from build123d import *

# Parameters (mm, degrees)
F0_W      = 2
F0_H      = 2
F1_DEPTH  = 3
F0_H_2    = 14
F0_W_2    = 14
F0_W_3    = 11
F2_DEPTH  = 2
F0_R      = 2.5
F3_DEPTH  = 4
F0_R_2    = 1.5
F0_R_3    = 0.95
F4_DEPTH  = 20
F5_DEPTH  = 17
F6_DEPTH  = 17
F7_DEPTH  = 17
F8_DEPTH  = 17
F0_W_4    = 6
F0_H_3    = 6
F9_DEPTH  = 2
F0_H_4    = 3
F10_DEPTH = 20
F0_W_5    = 3
F0_W_6    = 5
F0_W_7    = 1.1521804929
F0_H_5    = 5
F0_R_4    = 1.75
F0_R_5    = 1
F0_W_8    = 0.8478195071
F11_DEPTH = 2
F0_H_6    = 1
F12_DEPTH = 4
F0_W_9    = 2.5
F13_DEPTH = 4
F14_DEPTH = 2
F15_DEPTH = 2
F16_DEPTH = 0.5


# Not quite as in the source:
# - a feature names something its author has since deleted; it is built from what else it names


with BuildPart() as f1:
    # F0 (on Front) → F1 (new body)
    with BuildSketch(Plane.XZ):
        Polygon((16, 1), (16, 2), (2, 2), (1, 2), (-1, 2), (-1, 10), (-1, 16), (-2, 16), (-2, 2), (-4, 2), (-4, 16), (-5, 16), (-5, 2), (-16, 2), (-16, 1), (-5, 1), (-5, -1), (-16, -1), (-16, -2), (-5, -2), (-5, -16), (-4, -16), (-4, -2), (-2, -2), (-2, -16), (-1, -16), (-1, -2), (1, -2), (1, -16), (2, -16), (2, -2), (16, -2), (16, -1), (2, -1), (2, 1), align=None)
        with Locations((-3, 0)):
            Rectangle(F0_W, F0_H, mode=Mode.SUBTRACT)
        Rectangle(F0_W, F0_H, mode=Mode.SUBTRACT)
    extrude(amount=-F1_DEPTH)

    # F0 (on Front) → F2 (join)
    with BuildSketch(Plane.XZ):
        Polygon((16, 2), (16, 10.1685791543), (16, 11), (11, 11), (9.8478195071, 11), (9.8478195071, 10.2023985237), (9.8478195071, 10), (7.6956390142, 10), (7.6956390142, 7.9433578615), (7.6956390142, 6.0566421385), (7.6956390142, 4), (4.8478195071, 4), (2, 4), (2, 6.0566421385), (2, 7.9433578615), (2, 10), (-0.1521804929, 10), (-1, 10), (-1, 2), (1, 2), (2, 2), align=None)
        with Locations((-3, 9)):
            Rectangle(F0_W, F0_H_2)
        Polygon((16, -11), (16, -2), (2, -2), (2, -16), (11, -16), (11, -11), align=None)
        with Locations((9, 0)):
            Rectangle(F0_W_2, F0_H)
        with Locations((-10.5, 0)):
            Rectangle(F0_W_3, F0_H)
        Polygon((-11, -11), (-11, -16), (-5, -16), (-5, -2), (-16, -2), (-16, -11), align=None)
        with Locations((-3, -9)):
            Rectangle(F0_W, F0_H_2)
        with Locations((0, -9)):
            Rectangle(F0_W, F0_H_2)
        Polygon((-5, 2), (-5, 16), (-11, 16), (-11, 11), (-16, 11), (-16, 10), (-10, 10), (-10, 4), (-16, 4), (-16, 2), align=None)
        with Locations((-3, 0)):
            Rectangle(F0_W, F0_H)
        Rectangle(F0_W, F0_H)
    extrude(amount=-F2_DEPTH)

    # F0 (on Front) → F3 (join)
    with BuildSketch(Plane.XZ):
        Polygon((11, 11), (16, 11), (17, 11), (17, 13), (17, 14), (17, 17), (14, 17), (11, 17), (11, 16), align=None)
        with Locations((14, 14)):
            Circle(F0_R, mode=Mode.SUBTRACT)
        Polygon((-11, 16), (-11, 17), (-14, 17), (-17, 17), (-17, 14), (-17, 11), (-16, 11), (-11, 11), align=None)
        with Locations((-14, 14)):
            Circle(F0_R, mode=Mode.SUBTRACT)
        Polygon((-14, -17), (-11, -17), (-11, -16), (-11, -11), (-16, -11), (-17, -11), (-17, -14), (-17, -17), align=None)
        with Locations((-14, -14)):
            Circle(F0_R, mode=Mode.SUBTRACT)
        Polygon((17, -11), (16, -11), (11, -11), (11, -16), (11, -17), (14, -17), (17, -17), (17, -14), (17, -13), align=None)
        with Locations((14, -14)):
            Circle(F0_R, mode=Mode.SUBTRACT)
    extrude(amount=-F3_DEPTH)

    # F0 (on Front) → F4 (join)
    with BuildSketch(Plane.XZ):
        with Locations((14, 14)):
            Circle(F0_R)
        with Locations((14, 14)):
            Circle(F0_R_2, mode=Mode.SUBTRACT)
        with Locations((14, 14)):
            Circle(F0_R_2)
        with Locations((14, 14)):
            Circle(F0_R_3, mode=Mode.SUBTRACT)
        with Locations((-14, 14)):
            Circle(F0_R)
        with Locations((-14, 14)):
            Circle(F0_R_2, mode=Mode.SUBTRACT)
        with Locations((-14, 14)):
            Circle(F0_R_2)
        with Locations((-14, 14)):
            Circle(F0_R_3, mode=Mode.SUBTRACT)
        with Locations((-14, -14)):
            Circle(F0_R)
        with Locations((-14, -14)):
            Circle(F0_R_2, mode=Mode.SUBTRACT)
        with Locations((-14, -14)):
            Circle(F0_R_2)
        with Locations((-14, -14)):
            Circle(F0_R_3, mode=Mode.SUBTRACT)
        with Locations((14, -14)):
            Circle(F0_R)
        with Locations((14, -14)):
            Circle(F0_R_2, mode=Mode.SUBTRACT)
        with Locations((14, -14)):
            Circle(F0_R_2)
        with Locations((14, -14)):
            Circle(F0_R_3, mode=Mode.SUBTRACT)
    extrude(amount=-F4_DEPTH)

    # F0 (on Front) → F5 (cut)
    with BuildSketch(Plane.XZ):
        with Locations((-14, 14)):
            Circle(F0_R_2)
        with Locations((-14, 14)):
            Circle(F0_R_3, mode=Mode.SUBTRACT)
    extrude(amount=-F5_DEPTH, mode=Mode.SUBTRACT)

    # F0 (on Front) → F6 (cut)
    with BuildSketch(Plane.XZ):
        with Locations((14, 14)):
            Circle(F0_R_2)
        with Locations((14, 14)):
            Circle(F0_R_3, mode=Mode.SUBTRACT)
    extrude(amount=-F6_DEPTH, mode=Mode.SUBTRACT)

    # F0 (on Front) → F7 (cut)
    with BuildSketch(Plane.XZ):
        with Locations((-14, -14)):
            Circle(F0_R_2)
        with Locations((-14, -14)):
            Circle(F0_R_3, mode=Mode.SUBTRACT)
    extrude(amount=-F7_DEPTH, mode=Mode.SUBTRACT)

    # F0 (on Front) → F8 (cut)
    with BuildSketch(Plane.XZ):
        with Locations((14, -14)):
            Circle(F0_R_2)
        with Locations((14, -14)):
            Circle(F0_R_3, mode=Mode.SUBTRACT)
    extrude(amount=-F8_DEPTH, mode=Mode.SUBTRACT)

    # F0 (on Front) → F9 (join)
    with BuildSketch(Plane.XZ):
        with Locations((-13, 7)):
            Rectangle(F0_W_4, F0_H_3)
    extrude(amount=-F9_DEPTH)

    # F0 (on Front) → F10, piece 6 (join)
    with BuildSketch(Plane.XZ):
        with Locations((18, 18)):
            Rectangle(F0_W, F0_H)
        with Locations((18, 15.5)):
            Rectangle(F0_W, F0_H_4)
        with Locations((15.5, 18)):
            Rectangle(F0_W_5, F0_H)
        Polygon((9.8478195071, 17), (11, 17), (14, 17), (14, 19), (7.3478195071, 19), (7.3478195071, 17), align=None)
        with Locations((4.8478195071, 18)):
            Rectangle(F0_W_6, F0_H)
        Polygon((-0.1521804929, 17), (2.3478195071, 17), (2.3478195071, 19), (-14, 19), (-14, 17), (-11, 17), align=None)
        with Locations((-15.5, 18)):
            Rectangle(F0_W_5, F0_H)
        with Locations((-18, 18)):
            Rectangle(F0_W, F0_H)
        with Locations((-18, 15.5)):
            Rectangle(F0_W, F0_H_4)
        Polygon((-19, -14), (-17, -14), (-17, -11), (-17, -2), (-17, -1), (-17, 1), (-17, 2), (-17, 11), (-17, 14), (-19, 14), align=None)
        Polygon((17, 13), (17, 11), (17, 10), (19, 10), (19, 13), align=None)
        Polygon((17, -10), (17, -11), (17, -13), (19, -13), (19, -10), align=None)
        with Locations((18, -15.5)):
            Rectangle(F0_W, F0_H_4)
        with Locations((18, -18)):
            Rectangle(F0_W, F0_H)
        with Locations((15.5, -18)):
            Rectangle(F0_W_5, F0_H)
        Polygon((14, -17), (11, -17), (-11, -17), (-14, -17), (-14, -19), (14, -19), align=None)
        with Locations((-15.5, -18)):
            Rectangle(F0_W_5, F0_H)
        with Locations((-18, -18)):
            Rectangle(F0_W, F0_H)
        with Locations((-18, -15.5)):
            Rectangle(F0_W, F0_H_4)
    extrude(amount=-F10_DEPTH)

    # F0 (on Front) → F11 (join)
    with BuildSketch(Plane.XZ):
        with Locations((10.4239097536, 13.5)):
            Rectangle(F0_W_7, F0_H_5)
        with BuildLine():
            Line((7.6956390142, 7.9433578615), (7.6956390142, 10))
            Line((7.6956390142, 10), (4.8478195071, 10))
            ThreePointArc((4.8478195071, 10), (6.6042258404, 9.4320848653), (7.6956390142, 7.9433578615))
        make_face()
        with BuildLine():
            ThreePointArc((7.6956390142, 7.9433578615), (6.6042258404, 9.4320848653), (4.8478195071, 10))
            ThreePointArc((4.8478195071, 10), (3.0914131738, 9.4320848653), (2, 7.9433578615))
            Line((2, 7.9433578615), (2, 6.0566421385))
            ThreePointArc((2, 6.0566421385), (3.0914131738, 4.5679151347), (4.8478195071, 4))
            ThreePointArc((4.8478195071, 4), (6.6042258404, 4.5679151347), (7.6956390142, 6.0566421385))
            Line((7.6956390142, 6.0566421385), (7.6956390142, 7.9433578615))
        make_face()
        with Locations((4.8478195071, 7)):
            Circle(F0_R_4, mode=Mode.SUBTRACT)
        with BuildLine():
            Line((7.6956390142, 4), (7.6956390142, 6.0566421385))
            ThreePointArc((7.6956390142, 6.0566421385), (6.6042258404, 4.5679151347), (4.8478195071, 4))
            Line((4.8478195071, 4), (7.6956390142, 4))
        make_face()
        with Locations((4.8478195071, 7)):
            Circle(F0_R_4)
        with Locations((4.8478195071, 7)):
            Circle(F0_R_5, mode=Mode.SUBTRACT)
        with BuildLine():
            ThreePointArc((4.8478195071, 4), (3.0914131738, 4.5679151347), (2, 6.0566421385))
            Line((2, 6.0566421385), (2, 4))
            Line((2, 4), (4.8478195071, 4))
        make_face()
        with BuildLine():
            Line((4.8478195071, 10), (2, 10))
            Line((2, 10), (2, 7.9433578615))
            ThreePointArc((2, 7.9433578615), (3.0914131738, 9.4320848653), (4.8478195071, 10))
        make_face()
        with Locations((-0.5760902464, 13)):
            Rectangle(F0_W_8, F0_H_3)
    extrude(amount=-F11_DEPTH)



with BuildPart() as f10:
    # F0 (on Front) → F10 (new body)
    with BuildSketch(Plane.XZ):
        with Locations((18, 7.5)):
            Rectangle(F0_W, F0_H_4)
    extrude(amount=-F10_DEPTH)


with BuildPart() as f10b:
    # F0 (on Front) → F10, piece 2 (new body)
    with BuildSketch(Plane.XZ):
        with Locations((18, 3.5)):
            Rectangle(F0_W, F0_H_4)
    extrude(amount=-F10_DEPTH)


with BuildPart() as f10c:
    # F0 (on Front) → F10, piece 3 (new body)
    with BuildSketch(Plane.XZ):
        Polygon((19, 1), (17, 1), (17, 0), (17, -1), (19, -1), (19, 0), align=None)
    extrude(amount=-F10_DEPTH)


with BuildPart() as f10d:
    # F0 (on Front) → F10, piece 4 (new body)
    with BuildSketch(Plane.XZ):
        with Locations((18, -3.5)):
            Rectangle(F0_W, F0_H_4)
    extrude(amount=-F10_DEPTH)


with BuildPart() as f10e:
    # F0 (on Front) → F10, piece 5 (new body)
    with BuildSketch(Plane.XZ):
        with Locations((18, -7.5)):
            Rectangle(F0_W, F0_H_4)
    extrude(amount=-F10_DEPTH)


with BuildPart() as f1_1:
    add(f1.part)

    add(f10.part)  # F12 merges F10

    add(f10b.part)  # F12 merges F10b

    add(f10c.part)  # F12 merges F10c

    add(f10d.part)  # F12 merges F10d

    add(f10e.part)  # F12 merges F10e
    # F0 (on Front) → F12 (join)
    with BuildSketch(Plane.XZ):
        Polygon((16, 11), (16, 10.1685791543), (16, 2), (16, 1), (16, -1), (16, -2), (16, -11), (17, -11), (17, -10), (17, -9), (17, -6), (17, -5), (17, -2), (17, -1), (17, 0), (17, 1), (17, 2), (17, 5), (17, 6), (17, 9), (17, 10), (17, 11), align=None)
        with Locations((4.8478195071, 16.5)):
            Rectangle(F0_W_6, F0_H_6)
        Polygon((11, -16), (2, -16), (1, -16), (-1, -16), (-2, -16), (-4, -16), (-5, -16), (-11, -16), (-11, -17), (11, -17), align=None)
        Polygon((-2, 16), (-1, 16), (-0.1521804929, 16), (-0.1521804929, 17), (-11, 17), (-11, 16), (-5, 16), (-4, 16), align=None)
        Polygon((-16, 1), (-16, 2), (-16, 4), (-16, 10), (-16, 11), (-17, 11), (-17, 2), (-17, 1), (-17, -1), (-17, -2), (-17, -11), (-16, -11), (-16, -2), (-16, -1), align=None)
    extrude(amount=-F12_DEPTH)

    # F0 (on Front) → F13 (join)
    with BuildSketch(Plane.XZ):
        with Locations((10.4239097536, 16.5)):
            Rectangle(F0_W_7, F0_H_6)
        with Locations((8.5978195071, 16.5)):
            Rectangle(F0_W_9, F0_H_6)
        Polygon((2, 16), (2.3478195071, 16), (2.3478195071, 17), (-0.1521804929, 17), (-0.1521804929, 16), (1, 16), align=None)
    extrude(amount=-F13_DEPTH)

    # F0 (on Front) → F14 (cut)
    with BuildSketch(Plane.XZ):
        Polygon((2, 16), (2.3478195071, 16), (2.3478195071, 17), (-0.1521804929, 17), (-0.1521804929, 16), (1, 16), align=None)
    extrude(amount=-F14_DEPTH, mode=Mode.SUBTRACT)

    # F0 (on Front) → F15 (cut)
    with BuildSketch(Plane.XZ):
        with Locations((8.5978195071, 16.5)):
            Rectangle(F0_W_9, F0_H_6)
    extrude(amount=-F15_DEPTH, mode=Mode.SUBTRACT)

    # F0 (on Front) → F16 (cut)
    with BuildSketch(Plane.XZ):
        with Locations((4.8478195071, 7)):
            Circle(F0_R_4)
        with Locations((4.8478195071, 7)):
            Circle(F0_R_5, mode=Mode.SUBTRACT)
    extrude(amount=-F16_DEPTH, mode=Mode.SUBTRACT)


solid = f1_1.part
Geometry: final body of the model. Coordinates: model frame, mm. A direction names the side the tool comes from. Round coordinates to 2 decimals unless told otherwise and drop trailing zeros. Order: outer loops, then holes, each group sorted by start corner. A loop starts at its lowest first (then second) coordinate and runs counter-clockwise, first axis right, second up.
Q1. Access query for faces 3 (the face through (-3, 2.5, -2)), 4 (the face through (18, 10, 14)), 5 (the face through (1.1, 2, 16.5)), 6 (the face through (18, 20, -11)), 7 (the face through (19, 10, 11)). Directions: +Z, -Z, +X, -X, +Y, -Y. A direction counts if a zero-diameter tool reaches every point of the face in a straight line with its end or side. Return the directions, or none.
Result sheet:
face 3: +Y
face 4: +X, +Y, -Y
face 5: -Y
face 6: +Z, -Z, +X, -X, +Y
face 7: +Z, -Z, +X, +Y, -Y
Q2. Section A-A, the plane z = 7. Output: boundary loops of the cut face in (x, y), and give its area (3 significant figures).
Result sheet:
outline: (-19, 0) - (3.1, 0) - (3.1, 0.5) - (3.85, 0.5) - (3.85, 2) - (-1, 2) - (-1, 3) - (-2, 3) - (-2, 2) - (-4, 2) - (-4, 3) - (-5, 3) - (-5, 2) - (-16, 2) - (-16, 4) - (-17, 4) - (-17, 20) - (-19, 20) - close; (5.85, 0.5) - (6.6, 0.5) - (6.6, 0) - (19, 0) - (19, 20) - (17, 20) - (17, 4) - (16, 4) - (16, 2) - (5.85, 2) - close
area: 149 mm2
Q3. Pin query (flat end, axial travel): pin 1 (2.5 mm diameter, centred on x = 14, z = 14, fed in from -Y); pin 2 (0.8 mm diameter, centred on y = 1.5, z = -5.5, fed in from +X); pin 3 (1.6 mm diameter, centred on x = 0, z = 0, fed in from +Y). Return the tip coordinate at first contact, or that it passes through.
Result sheet:
pin 1: stops at y = 17
pin 2: stops at x = 17
pin 3: stops at y = 2
Q4. Section C-C, the plane x = 10.5. Output: boundary loops of the cut face in (y, z).
Result sheet:
outline: (0, -19) - (20, -19) - (20, -17) - (4, -17) - (4, -16) - (2, -16) - (2, -2) - (3, -2) - (3, -1) - (2, -1) - (2, 1) - (3, 1) - (3, 2) - (2, 2) - (2, 16) - (4, 16) - (4, 17) - (20, 17) - (20, 19) - (0, 19) - close
Q5. Material intervals for probe 1 along X at (y, z) = (4.5, -16); probe 2 along Z at (x, y) = (-14, 18.25), sorted ascending.
Result sheet:
probe 1: x = -19 to -17, -15.5 to -12.5, 12.5 to 15.5, 17 to 19
probe 2: z = -19 to -17, -16.5 to -14.95, -13.05 to -11.5, 11.5 to 13.05, 14.95 to 16.5, 17 to 19
Q6. Section B-B, the plane y = 12.5. Give the number of separate pieces and of enclosed holes in the cut face, and give its area (3 significant figures).
Result sheet:
separate pieces: 12
enclosed holes: 4
area: 322 mm2
Q7. Section D-D, the plane z = -6.5. Output: boundary loops of the cut face in (x, y), and give its area (3 significant figures).
Result sheet:
outline: (-19, 0) - (19, 0) - (19, 20) - (17, 20) - (17, 4) - (16, 4) - (16, 2) - (2, 2) - (2, 3) - (1, 3) - (1, 2) - (-1, 2) - (-1, 3) - (-2, 3) - (-2, 2) - (-4, 2) - (-4, 3) - (-5, 3) - (-5, 2) - (-16, 2) - (-16, 4) - (-17, 4) - (-17, 20) - (-19, 20) - close
area: 155 mm2
Q8. Mould query, pull axis Z, two halves, no side actions, for faces 1 (the face through (19, 10, -17)), 2 (the face through (1, 2.5, 0)). Classes: released by +Z, released by -Z, zero draft, split by the parting line, or undercut.
Result sheet:
face 1: zero draft
face 2: undercut
